```python
from build123d import *

# Parameters (mm, degrees)
SKETCH13_W                   = 111.84
SKETCH13_H                   = 111.84
BASE_FLANGE2_DEPTH           = 5
EDGE_FLANGE1_STRIP_W         = 21.4732
EDGE_FLANGE1_STRIP_H         = 5
EDGE_FLANGE1_STRIP_CUT_DEPTH = 111.84
EDGE_FLANGE1_DEPTH           = 111.84
EDGE_FLANGE2_STRIP_W         = 21.4732
EDGE_FLANGE2_STRIP_H         = 5
EDGE_FLANGE2_STRIP_CUT_DEPTH = 111.84
EDGE_FLANGE2_DEPTH           = 111.84
SKETCH25_R                   = 5
CUT_EXTRUDE1_DEPTH           = 209.139184211
SKETCH27_W                   = 5
SKETCH27_H                   = 5
BOSS_EXTRUDE3_DEPTH          = 35.342
SKETCH28_W                   = 5
SKETCH28_H                   = 5
BOSS_EXTRUDE1_DEPTH          = 36.5
BOSS_EXTRUDE2_DEPTH          = 5
SKETCH40_R                   = 5.2455
BOSS_EXTRUDE7_DEPTH          = 31.3


# Sheet-metal steps are written as plain solids
with BuildPart() as part:
    # Sketch13 → Base-Flange2 (new body)
    with BuildSketch(Plane.XY):
        with Locations((55.92, 55.92)):
            Rectangle(SKETCH13_W, SKETCH13_H)
    extrude(amount=-BASE_FLANGE2_DEPTH)

    # Edge-Flange1 strip (across the edge) → Edge-Flange1 strip cut (cut)
    with BuildSketch(Plane.XZ.offset(-111.84)):
        with Locations((-5, -2.5)):
            Rectangle(EDGE_FLANGE1_STRIP_W, EDGE_FLANGE1_STRIP_H)
    extrude(amount=EDGE_FLANGE1_STRIP_CUT_DEPTH, mode=Mode.SUBTRACT)

    # Edge-Flange1 section (across the edge) → Edge-Flange1 (add)
    with BuildSketch(Plane.XZ.offset(-111.84)):
        with BuildLine():
            Line((0, 0.7366), (0, 135.298))
            Line((0, 135.298), (5, 135.298))
            Line((5, 135.298), (5, 0.7366))
            ThreePointArc((5, 0.7366), (5.215745145, 0.215745145), (5.7366, 0))
            Line((5.7366, 0), (5.7366, -5))
            ThreePointArc((5.7366, -5), (1.680211239, -3.319788761), (0, 0.7366))
        make_face()
    extrude(amount=EDGE_FLANGE1_DEPTH)

    # Edge-Flange2 strip (across the edge) → Edge-Flange2 strip cut (cut)
    with BuildSketch(Plane(origin=(111.84, 0, 0), x_dir=(-1, 0, 0), z_dir=(0, 1, 0))):
        with Locations((-5, -2.5)):
            Rectangle(EDGE_FLANGE2_STRIP_W, EDGE_FLANGE2_STRIP_H)
    extrude(amount=EDGE_FLANGE2_STRIP_CUT_DEPTH, mode=Mode.SUBTRACT)

    # Edge-Flange2 section (across the edge) → Edge-Flange2 (add)
    with BuildSketch(Plane(origin=(111.84, 0, 0), x_dir=(-1, 0, 0), z_dir=(0, 1, 0))):
        with BuildLine():
            Line((0, 0.7366), (0, 135.298))
            Line((0, 135.298), (5, 135.298))
            Line((5, 135.298), (5, 0.7366))
            ThreePointArc((5, 0.7366), (5.215745145, 0.215745145), (5.7366, 0))
            Line((5.7366, 0), (5.7366, -5))
            ThreePointArc((5.7366, -5), (1.680211239, -3.319788761), (0, 0.7366))
        make_face()
    extrude(amount=EDGE_FLANGE2_DEPTH)

    # Sketch25 → Cut-Extrude1 (cut, through all)
    with BuildSketch(Plane.XY):
        with Locations((30.7366, 91.84)):
            Circle(SKETCH25_R)
        with Locations(Location((81.1034, 91.84, 0), (0, 0, 180))):
            Circle(SKETCH25_R)
    extrude(amount=-CUT_EXTRUDE1_DEPTH, mode=Mode.SUBTRACT)

    # Sketch27 → Boss-Extrude3 (add)
    with BuildSketch(Plane(origin=(5, 0, 0), x_dir=(0, 0, -1), z_dir=(1, 0, 0))):
        with Locations((-70.5, 22)):
            Rectangle(SKETCH27_W, SKETCH27_H)
    extrude(amount=BOSS_EXTRUDE3_DEPTH)

    # Sketch28 → Boss-Extrude1 (add)
    with BuildSketch(Plane.ZY.offset(-106.84)):
        with Locations((70.5, 22)):
            Rectangle(SKETCH28_W, SKETCH28_H)
    extrude(amount=BOSS_EXTRUDE1_DEPTH)

    # Sketch29 → Boss-Extrude2 (add)
    with BuildSketch(Plane(origin=(0, 24.5, 0), x_dir=(1, 0, 0), z_dir=(0, 1, 0))):
        with BuildLine():
            Line((45.436988134, -73), (47.484648624, -73))
            ThreePointArc((47.484648624, -73), (57.888494067, -59.8), (68.29233951, -73))
            Line((68.29233951, -73), (70.34, -73))
            ThreePointArc((70.34, -73), (57.888494067, -57.8), (45.436988134, -73))
        make_face()
    extrude(amount=-BOSS_EXTRUDE2_DEPTH)

    # Sketch40 → Boss-Extrude7 (add)
    with BuildSketch(Plane(origin=(5, 0, 0), x_dir=(0, 0, -1), z_dir=(1, 0, 0))):
        with Locations((-105, 75.186)):
            Circle(SKETCH40_R)
    extrude(amount=BOSS_EXTRUDE7_DEPTH)


solid = part.part
```
For this review, take the finished solid that the model builds, in its own axes (mm). A direction names the side the tool comes from. Round coordinates to 2 decimals unless told otherwise and drop trailing zeros. Order: outer loops, then holes, each group sorted by start corner. A loop starts at its lowest first (then second) coordinate and runs counter-clockwise, first axis right, second up. Notation, with made-up numbers: (5, -29) -> (53, -29) arc R12 ccw to (53, -7) -> close; hole circle Ø6 at (71, 50.5). An arc over 180 degrees is marked (long way). Use a Markdown table: item, result.
Item 1: Take a section at C-C (x = 96). State the section outline as (y, z) points.
Resolved:
| item | result |
|---|---|
| outline | (0, -5) -> (111.84, -5) -> (111.84, 0) -> (0, 0) -> close; (19.5, 68) -> (24.5, 68) -> (24.5, 73) -> (19.5, 73) -> close |
Item 2: For line 1 along Z through (x, y) = (93, 23); line 2 along X through (y, z) = (99, 65.5); line 3 along X through (y, z) = (91, -3), list the stretches that pass through material, from the lowest coordinate up. Write a range as [from, to].
Resolved:
| item | result |
|---|---|
| line 1 | z = [-5, 0], [68, 73] |
| line 2 | x = [0, 5], [106.84, 111.84] |
| line 3 | x = [1.38, 25.81], [35.67, 76.17], [86.03, 110.46] |
Item 3: Take a section at A-A (z = 70.5). State the section outline as (x, y) points, plus the area to 3 significant figures.
Resolved:
| item | result |
|---|---|
| outline | (0, 0) -> (5, 0) -> (5, 19.5) -> (40.34, 19.5) -> (40.34, 24.5) -> (5, 24.5) -> (5, 111.84) -> (0, 111.84) -> close; (45.19, 19.5) -> (47.19, 19.5) -> (47.19, 24.5) -> (45.19, 24.5) -> close; (68.59, 19.5) -> (106.84, 19.5) -> (106.84, 0) -> (111.84, 0) -> (111.84, 111.84) -> (106.84, 111.84) -> (106.84, 24.5) -> (68.59, 24.5) -> close |
| area | 1,500 mm² |
Item 4: Take a section at D-D (z = 105). State the section outline as (x, y) points, plus the area to 3 significant figures.
Resolved:
| item | result |
|---|---|
| outline | (0, 0) -> (5, 0) -> (5, 69.94) -> (36.3, 69.94) -> (36.3, 80.43) -> (5, 80.43) -> (5, 111.84) -> (0, 111.84) -> close; (106.84, 0) -> (111.84, 0) -> (111.84, 111.84) -> (106.84, 111.84) -> close |
| area | 1,450 mm² |
Item 5: Machinability: for faces 4 (the flat face through (89, 22, 68)), 5 (the flat face through (87, 22, 73)), 6 (the cylindrical face through (20.431, 80.387, 105.683)), which of the approach directions +Z, -Z, +X, -X, +Y, -Y give a long, thin tool a straight path to every point of the face, cutting with its end or side? Answer none if there is none.
Resolved:
| item | result |
|---|---|
| face 4 | +Y, -Y |
| face 5 | +Z, +Y, -Y |
| face 6 | none |
Item 6: For pin 1 (1.5 mm diameter, centred on x = 53.5, y = 62.5, fed in from +Z); pin 2 (7.5 mm diameter, centred on x = 75.5, z = 65, fed in from -Y); pin 3 (1.5 mm diameter, centred on x = 87, y = 21.5, fed in from +Z); pin 4 (9 mm diameter, centred on x = 30.74, y = 91.84, fed in from -Z), all flat-tipped, find the tip position at first contact; note any pin that passes through.
Resolved:
| item | result |
|---|---|
| pin 1 | stops at z = 0 |
| pin 2 | stops at y = 19.5 |
| pin 3 | stops at z = 73 |
| pin 4 | passes through |
Item 7: Draft analysis for pull direction X (two halves, no side actions). For faces 1 (the flat face through (22, 24.5, 71)), 2 (the cylindrical face through (1.725, 56.703, -3.364)), 3 (the flat face through (2, 57, 135.298)), state which applies: +X half, -X half, draft (parallel to the pull), parting line (faces both ways), or undercut.
Resolved:
| item | result |
|---|---|
| face 1 | undercut |
| face 2 | -X half |
| face 3 | draft |
Item 8: Take a section at B-B (y = 91.84). State the section outline as (x, z) points, plus the area to 3 significant figures.
Resolved:
| item | result |
|---|---|
| outline | (0, 0.74) arc R5.74 ccw to (5.74, -5) -> (25.74, -5) -> (25.74, 0) -> (5.74, 0) arc R0.74 cw to (5, 0.74) -> (5, 135.3) -> (0, 135.3) -> close; (35.74, -5) -> (76.1, -5) -> (76.1, 0) -> (35.74, 0) -> close; (86.1, -5) -> (106.1, -5) arc R5.74 ccw to (111.84, 0.74) -> (111.84, 135.3) -> (106.84, 135.3) -> (106.84, 0.74) arc R0.74 cw to (106.1, 0) -> (86.1, 0) -> close |
| area | 1,800 mm² |
